Design review of the part built by this model. Coordinates are the model's own, in mm. A direction names the side the tool comes from. Give positions to 0.01 mm unless a question says otherwise; leave off trailing zeros. Loops run counter-clockwise (first coordinate to the right, second up) from the corner with the lowest first, then second, coordinate; pieces in that order, holes last. Notation, with made-up numbers: M 50,84 L 87,84 A17 cw 87,91 Z; hole C -2,-14.5 d1. An arc over 180 degrees is marked long. Use one line per item in the form item = value. Start each with the question number.
from build123d import *

# Parameters (mm, degrees)
SKETCH1_R               = 7.1374
BOSS_EXTRUDE1_DEPTH     = 23.5966
CHAMFER1_SIZE           = 0.254
CHAMFER2_SIZE           = 0.254
SKETCH2_R               = 4.7625
CUT_EXTRUDE1_DEPTH      = 7.1755
SKETCH3_R               = 6.35
CUT_EXTRUDE2_DEPTH      = 28.513757958
CUT_EXTRUDE3_REACH      = 27.665
CUT_EXTRUDE3_END_RADIUS = 4.7625
SKETCH4_R               = 3.175


with BuildPart() as part:
    # Sketch1 → Boss-Extrude1 (new body)
    with BuildSketch(Plane(origin=(0, 0, 0), x_dir=(1, 0, 0), z_dir=(0, 1, 0))):
        with Locations(Location((0, 0, 0), (0, 0, 90))):
            Circle(SKETCH1_R)
    extrude(amount=BOSS_EXTRUDE1_DEPTH)

    # Chamfer1
    chamfer1_edges = [part.edges().sort_by_distance(p)[0] for p in [
        (0, 0, 7.1374),
    ]]
    chamfer(chamfer1_edges, length=CHAMFER1_SIZE)

    # Chamfer2
    chamfer2_edges = [part.edges().sort_by_distance(p)[0] for p in [
        (0, 23.5966, 7.1374),
    ]]
    chamfer(chamfer2_edges, length=CHAMFER2_SIZE)

    # Sketch2 → Cut-Extrude1 (cut, symmetric)
    with BuildSketch(Plane.XY):
        with Locations(Location((0, 11.7983, 0), (0, 0, 89.999999998))):
            Circle(SKETCH2_R)
    extrude(amount=CUT_EXTRUDE1_DEPTH, both=True, mode=Mode.SUBTRACT)

    # Sketch3 → Cut-Extrude2 (cut, through all)
    with BuildSketch(Plane.XY.offset(5.08)):
        with Locations((0, 11.7983)):
            Circle(SKETCH3_R)
    cut_extrude2 = extrude(amount=CUT_EXTRUDE2_DEPTH, mode=Mode.SUBTRACT)

    # Mirror1: Cut-Extrude2 across plane
    add(cut_extrude2.mirror(Plane.XY), mode=Mode.SUBTRACT)

    # Cut-Extrude3: up to this cylinder (the profile starts outside it)
    cut_extrude3_end = Plane(origin=(0, 11.7983, 0), z_dir=(0, 0, 1)) * Cylinder(CUT_EXTRUDE3_END_RADIUS, 65.855, mode=Mode.PRIVATE)
    # Sketch4 → Cut-Extrude3 (cut, up to the surface)
    with BuildSketch(Plane.XZ, mode=Mode.PRIVATE) as cut_extrude3_sk1:
        with Locations(Location((0, 0, 0), (0, 0, 270))):
            Circle(SKETCH4_R)
    cut_extrude3_tool1 = extrude(cut_extrude3_sk1.sketch, amount=-CUT_EXTRUDE3_REACH, mode=Mode.PRIVATE) - cut_extrude3_end
    add(cut_extrude3_tool1.solids().sort_by_distance((0, 0, 0))[0], mode=Mode.SUBTRACT)


solid = part.part
Q1. The part is to be moulded in two halves that separate along X. For faces 5 (the cylindrical face through (-6.018, 11.637, -3.837)), 6 (the flat face through (0, 23.597, 0)), 7 (the cylindrical face through (-0.08, 5.45, -5.87)), say which applies: pulls with the +X half, pulls with the -X half, needs draft (parallel to the pull), parting line crosses it, or undercut.
Q2. Take a section at A-A on x = 0. Give the boundary of the cut face in (y, z) (3 decimals), plus the area to 3 significant figures.
Q3. Take a section at D-D on y = 1.5. Give the boundary of the cut face in (x, z) (3 decimals), plus the area to 3 significant figures.
Q4. Wall thickness on probe 1 along X at (y, z) = (6.5, 0) (3 decimals); probe 2 along Z at (x, y) = (5, 12); probe 3 along X at (y, z) = (11.5, -1): over which ranges is each line inside the solid? List them lowest first.
Q5. Take a section at B-B on y = 9.5. Give the boundary of the cut face in (x, z), plus the area to 3 significant figures.
Q6. For faces 1 (the cylindrical face through (0.081, 18.148, -5.866)), 2 (the cylindrical face through (-1.43, 16.34, 0.07)), 3 (the cylindrical face through (0.95, 4.07, -3.03)), 4 (the flat face through (-1, 17, 5.08)), list the 3-axis set-ups (+Z, -Z, +X, -X, +Y, -Y) from which the entire face can be reached by the end or side of a thin tool; tool diameter is ignored.
Q7. Clearance check with flat-ended pins moving along their axes: pin 1 Ø8 at (x, y) = (3.5, 9.5) entering from -Z; pin 2 Ø4 at (y, z) = (17.5, -2.5) entering from +X; pin 3 Ø1 at (x, y) = (-1.5, 3.5) entering from -Z. State where each tip first meets the part, or that it passes through.
Response values:
q1.face_5 = parting line crosses it
q1.face_6 = needs draft
q1.face_7 = undercut
q2.outline = M 0,-6.883 L 0.254,-7.137 L 5.448,-7.137 L 5.448,-5.08 L 7.036,-5.08 L 7.036,-3.175 L 0,-3.175 Z; M 0,3.175 L 7.036,3.175 L 7.036,5.08 L 5.448,5.08 L 5.448,7.137 L 0.254,7.137 L 0,6.883 Z; M 16.561,-5.08 L 18.148,-5.08 L 18.148,-7.137 L 23.343,-7.137 L 23.597,-6.883 L 23.597,6.883 L 23.343,7.137 L 18.148,7.137 L 18.148,5.08 L 16.561,5.08 Z
q2.area = 143 mm^2
q3.outline = C 0,0 d14.275; hole C 0,0 d6.35
q3.area = 128 mm^2
q4.probe_1 = -7.137 to -3.175, 3.175 to 7.137
q4.probe_2 = -5.08 to 5.08
q4.probe_3 = -7.07 to -4.75, 4.75 to 7.07
q5.outline = M -5.01,-5.08 L -4.17,-5.08 L -4.17,5.08 L -5.01,5.08 A7.14 ccw Z; M 4.17,-5.08 L 5.01,-5.08 A7.14 ccw 5.01,5.08 L 4.17,5.08 Z
q5.area = 46.9 mm^2
q6.face_1 = -Z
q6.face_2 = +Z, -Z
q6.face_3 = -Y
q6.face_4 = +Z
q7.pin_1 = -6.84
q7.pin_2 = 7.12
q7.pin_3 = -7.07
